```python
from build123d import *

# Parameters (mm, degrees)
F3_W     = 20
F3_H     = 80
F4_DEPTH = 500
F6_D     = 17.5
F6_DEPTH = 40
F6_TIP   = 5.2575304165
F7_DEPTH = 40
F8_DEPTH = 35
F9_DEPTH = 35


# Not quite as in the source:
# - a feature names something its author has since deleted; it is built from what else it names


with BuildPart() as f4:
    # F3 (on Right) → F4 (new body, symmetric)
    with BuildSketch(Plane.YZ):
        with BuildLine():
            ThreePointArc((-4.2945303673, -84.5), (-3.7087439297, -85.9142135624), (-2.2945303673, -86.5))
            Line((-2.2945303673, -86.5), (33.7054696327, -86.5))
            ThreePointArc((33.7054696327, -86.5), (35.1196831951, -85.9142135624), (35.7054696327, -84.5))
            Line((35.7054696327, -84.5), (35.7054696327, 11.5))
            ThreePointArc((35.7054696327, 11.5), (35.1196831951, 12.9142135624), (33.7054696327, 13.5))
            Line((33.7054696327, 13.5), (-2.2945303673, 13.5))
            ThreePointArc((-2.2945303673, 13.5), (-3.7087439297, 12.9142135624), (-4.2945303673, 11.5))
            Line((-4.2945303673, 11.5), (-4.2945303673, -84.5))
        make_face()
        with Locations((15.7054696327, -36.5)):
            Rectangle(F3_W, F3_H, mode=Mode.SUBTRACT)
    extrude(amount=F4_DEPTH, both=True)

    # F6
    with Locations(Plane.XZ.offset(4.2945303673)):
        with Locations((450, -36.2195856869), (0, -36.2195856869), (-450, -36.5)):
            Hole(F6_D / 2, depth=F6_DEPTH)
            with Locations((0, 0, -(F6_DEPTH + F6_TIP / 2))):  # 118° drill point
                Cone(0, F6_D / 2, F6_TIP, mode=Mode.SUBTRACT)

    # F5 (on face) → F7 (cut)
    with BuildSketch(Plane.XZ.offset(4.2945303673)):
        with BuildLine():
            ThreePointArc((-500, -36.5), (-490, -6.5), (-464, 11.5))
            Line((-464, 11.5), (-500, 11.5))
            Line((-500, 11.5), (-500, -36.5))
        make_face()
        with BuildLine():
            ThreePointArc((-464, -84.5), (-490, -66.5), (-500, -36.5))
            Line((-500, -36.5), (-500, -84.5))
            Line((-500, -84.5), (-464, -84.5))
        make_face()
        with BuildLine():
            Line((500, 11.5), (464, 11.5))
            ThreePointArc((464, 11.5), (490, -6.5), (500, -36.5))
            Line((500, -36.5), (500, 11.5))
        make_face()
        with BuildLine():
            Line((500, -84.5), (500, -36.5))
            ThreePointArc((500, -36.5), (490, -66.5), (464, -84.5))
            Line((464, -84.5), (500, -84.5))
        make_face()
    extrude(amount=-F7_DEPTH, mode=Mode.SUBTRACT)

    # F8 (cut): faces of the model
    f8_faces = [f4.faces().sort_by_distance(p)[0] for p in [
        (-500, 15.7054696327, 12.4878664624),
        (-500, 15.7054696327, -85.4878664624),
    ]]
    extrude(f8_faces, amount=-F8_DEPTH, mode=Mode.SUBTRACT)

    # F9 (cut): faces of the model
    f9_faces = [f4.faces().sort_by_distance(p)[0] for p in [
        (500, 15.7054696327, -85.4878664624),
        (500, 15.7054696327, 12.4878664624),
    ]]
    extrude(f9_faces, amount=-F9_DEPTH, mode=Mode.SUBTRACT)


solid = f4.part
```
Work out the finished part from the listing and answer in its coordinate system (mm). A direction names the side the tool comes from. Give positions to 0.01 mm unless a question says otherwise; leave off trailing zeros. Write each loop counter-clockwise with the first axis right and the second up, starting at its lowest first coordinate (ties: lowest second). Pieces come first, ordered by that corner, then holes. Notation, with made-up numbers: (-36, 69) - (-14, 69) arc R20 ccw to (-14, 94) - close; hole circle Ø11 at (88, -35). An arc over 180 degrees is marked (long way). Use one line per item in the form item = value.
1. A cutting plane is placed at C-C (x = 17.5). Write down the section's boundary in (y, z), and give its area (3 significant figures).
Filled in:
outline = (-4.29, -84.5) arc R2 ccw to (-2.29, -86.5) - (33.71, -86.5) arc R2 ccw to (35.71, -84.5) - (35.71, 11.5) arc R2 ccw to (33.71, 13.5) - (-2.29, 13.5) arc R2 ccw to (-4.29, 11.5) - close; hole (5.71, -76.5) - (25.71, -76.5) - (25.71, 3.5) - (5.71, 3.5) - close
area = 2,400 mm^2
2. A cutting plane is placed at A-A (x = 450). Write down the section's boundary in (y, z).
Filled in:
outline = (-4.29, -84.5) arc R2 ccw to (-2.29, -86.5) - (33.71, -86.5) arc R2 ccw to (35.71, -84.5) - (35.71, -44.97) - (25.71, -44.97) - (25.71, -76.5) - (5.71, -76.5) - (5.71, -44.97) - (-4.29, -44.97) - close; (-4.29, -27.47) - (5.71, -27.47) - (5.71, 3.5) - (25.71, 3.5) - (25.71, -27.47) - (35.71, -27.47) - (35.71, 11.5) arc R2 ccw to (33.71, 13.5) - (-2.29, 13.5) arc R2 ccw to (-4.29, 11.5) - close
3. For faces 1 (the face through (7, 35.705, -48)), 2 (the face through (7, 16, -76.5)), determine the directions among +Z, -Z, +X, -X, +Y, -Y from which every point of the face is accessible in a straight line to the end or side of a thin tool.
Filled in:
face_1 = +Z, -Z, +X, -X, +Y
face_2 = +X, -X
4. A cutting plane is placed at B-B (y = 12). Write down the section's boundary in (x, z), and give its area (3 significant figures).
Filled in:
outline = (-480, -76.5) arc R50 ccw to (-464, -84.5) - (-465, -84.5) - (-465, -86.5) - (465, -86.5) - (465, -84.5) - (464, -84.5) arc R50 ccw to (480, -76.5) - close; (-480, 3.5) - (480, 3.5) arc R50 ccw to (464, 11.5) - (465, 11.5) - (465, 13.5) - (-465, 13.5) - (-465, 11.5) - (-464, 11.5) arc R50 ccw to start
area = 18,900 mm^2
5. Determine the mould class of faces 3 (the face through (441.917, 30.775, -39.571)), 4 (the face through (7, -4.295, -25)), 5 (the face through (7, 5.705, -46)) for opening direction Y: released by +Y, released by -Y, zero draft, split by the parting line, or undercut.
Filled in:
face_3 = zero draft
face_4 = released by -Y
face_5 = undercut
6. Consider L1, parallel to Y at x = -262.5, z = -59; L2, parallel to Z at x = 0, y = 31; L3, parallel to Z at x = -450, y = 2. Determine where each line is inside the solid, lowest interval first.
Filled in:
L1 = -4.29 to 5.71, 25.71 to 35.71
L2 = -86.5 to -44.97, -27.47 to 13.5
L3 = -86.5 to -45.25, -27.75 to 13.5
7. A cutting plane is placed at D-D (z = -56.5). Write down the section's boundary in (x, y).
Filled in:
outline = (-495.83, -4.29) - (495.83, -4.29) - (495.83, 5.71) - (-495.83, 5.71) - close; (-495.83, 25.71) - (495.83, 25.71) - (495.83, 35.71) - (-495.83, 35.71) - close
8. Each of these flat-tipped pins is pushed along its axis until it touches: pin 1 Ø12 at (y, z) = (28, -23) entering from -X; pin 2 Ø1 at (y, z) = (20, -85.5) entering from -X; pin 3 Ø12 at (y, z) = (25, -66) entering from -X. Where does it stop, or does it pass through?
Filled in:
pin_1 = -499.43
pin_2 = -465
pin_3 = -494.11
